Source: CAD feature listing. Evaluate the final solid. Frame: model axes, mm. Face numbers are marked on the shaded views. A direction names the side the tool comes from. Coordinates: 2 decimals unless noted, no trailing zeros. Order: outer loops, then holes, each group sorted by start corner. A loop starts at its lowest first (then second) coordinate and runs counter-clockwise, first axis right, second up. Notation, with made-up numbers: (-34.5, 12.5) -> (7.5, 12.5) arc R33 ccw to (7.5, 47.5) -> close; hole circle Ø3 at (16, 37.5). An arc over 180 degrees is marked (long way). Put each result on its own line as item: value.
from build123d import *

# Parameters (mm, degrees)
F0_R           = 9
F1_DEPTH       = 1
F3_DEPTH       = 3
F4_R           = 9
F5_DEPTH       = 6
F7_D           = 3.4
F7_DEPTH       = 6
F7_CSINK_D     = 6
F7_CSINK_ANGLE = 100
F7_TIP         = 1.0214630523


# Not quite as in the source:
# - a fillet or chamfer that OpenCascade refuses, or shapes differently, is made with other operations: its cross-section is extruded or revolved along the edge and cut away or added


with BuildPart() as f1:
    # F0 (on Top) → F1 (new body)
    with BuildSketch(Plane.XY):
        Circle(F0_R)
    extrude(amount=F1_DEPTH)

    # F2 (on face) → F3 (join)
    with BuildSketch(Plane.XY.offset(1)):
        with BuildLine():
            Line((2.9, 5.6743157806), (2.9, 1.6743157806))
            Line((2.9, 1.6743157806), (2.9, -1.6743157806))
            Line((2.9, -1.6743157806), (0, -3.3486315613))
            Line((0, -3.3486315613), (-2.9, -1.6743157806))
            Line((-2.9, -1.6743157806), (-2.9, 1.6743157806))
            Line((-2.9, 1.6743157806), (-2.9, 5.6743157806))
            Line((-2.9, 5.6743157806), (-5.2062932022, 7.3412881086))
            ThreePointArc((-5.2062932022, 7.3412881086), (-4.1317890302, -7.995518708), (9, 0))
            ThreePointArc((9, 0), (7.995518708, 4.1317890302), (5.2062932022, 7.3412881086))
            Line((5.2062932022, 7.3412881086), (2.9, 5.6743157806))
        make_face()
    extrude(amount=F3_DEPTH)

    # F4 (on face) → F5 (join)
    with BuildSketch(Plane.XY.offset(4)):
        Circle(F4_R)
    extrude(amount=F5_DEPTH)

    # F6: fillet of radius 9 on 1 edges, made by hand

    # F6_s1 → F6_t2 (revolve, cut)
    with BuildSketch(Plane.XZ):
        with BuildLine():
            ThreePointArc((9, 1), (6.3639610307, 7.3639610307), (0, 10))
            Line((0, 10), (9, 10))
            Line((9, 10), (9, 1))
        make_face()
    revolve(axis=Axis((0, 0, 10), (0, 0, 1)), mode=Mode.SUBTRACT)

    # F7
    with Locations(Plane(origin=(0, 0, 0), x_dir=(1, 0, 0), z_dir=(0, 0, -1))):
        with Locations((0, 0)):
            CounterSinkHole(F7_D / 2, F7_CSINK_D / 2, depth=F7_DEPTH, counter_sink_angle=F7_CSINK_ANGLE)
            with Locations((0, 0, -(F7_DEPTH + F7_TIP / 2))):  # 118° drill point
                Cone(0, F7_D / 2, F7_TIP, mode=Mode.SUBTRACT)


solid = f1.part
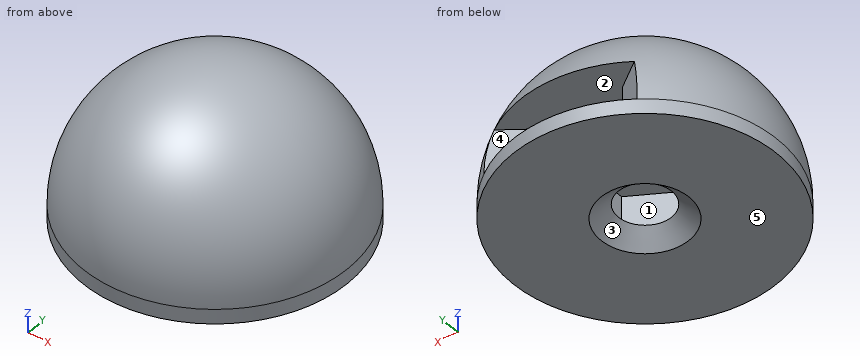
1. Cut plane D-D on z = 7.5. Output: boundary loops of the cut face in (x, y), plus the area to 3 significant figures.
Numbers:
outline: circle Ø12.45 at (0, 0)
area: 122 mm2
2. Pull-direction query (Y, two-part tool) for the marked faces 1, 2 and 3; classes: pulls with the +Y half, pulls with the -Y half, needs draft (parallel to the pull), parting line crosses it, or undercut.
Numbers:
face 1: pulls with the +Y half
face 2: needs draft
face 3: undercut
3. Cut plane A-A on x = -5.75. Output: boundary loops of the cut face in (y, z), plus the area to 3 significant figures.
Numbers:
outline: (-6.92, 0) -> (6.92, 0) -> (6.92, 1) arc R6.92 ccw to (-6.92, 1) -> close
area: 89.1 mm2
4. Set-up query: the marked faces 4 and 5. Return all of +Z, -Z, +X, -X, +Y, -Y with unobstructed straight access to the full face (end or side cutting, diameter ignored); none if empty.
Numbers:
face 4: +Y
face 5: -Z, +X, -X, +Y, -Y
5. First-contact query: pin 1 (3 mm diameter, centred on x = -2, y = 4, fed in from +Z); pin 2 (0.9 mm diameter, centred on y = 1, z = 2.5, fed in from -X); pin 3 (1.5 mm diameter, centred on x = 5, z = 1.5, fed in from +Y). Flat tips, straight axial feed; report the tip coordinate or a pass-through.
Numbers:
pin 1: stops at z = 9.5
pin 2: stops at x = -8.9
pin 3: stops at y = 7.83
6. Ray query, line 1 along Z through (x, y) = (-4.25, 7.5); line 2 along Y through (x, z) = (0, 4.6); line 3 along Y through (x, z) = (0, 5.5). Return the intervals inside material, ascending.
Numbers:
line 1: z = 0 to 1
line 2: y = -8.25 to -1.7, 1.7 to 8.25
line 3: y = -7.79 to -1.7, 1.7 to 7.79
7. Cut plane B-B on y = -6. Output: boundary loops of the cut face in (x, z).
Numbers:
outline: (-6.71, 0) -> (6.71, 0) -> (6.71, 1) arc R6.71 ccw to (-6.71, 1) -> close
8. Cut plane C-C on z = 9.5. Output: boundary loops of the cut face in (x, y), plus the area to 3 significant figures.
Numbers:
outline: circle Ø5.92 at (0, 0)
area: 27.5 mm2
